Source: three-view drawing plus pictorial views. Frame: mm from the lowest corner of the part. Give positions to 0.01 mm unless a question says otherwise; leave off trailing zeros. Loops run counter-clockwise (first coordinate to the right, second up) from the corner with the lowest first, then second, coordinate; pieces in that order, holes last. Notation, with made-up numbers: (14.25, 47) -> (68.25, 47) arc R16 cw to (68.25, 52) -> close; hole circle Ø1 at (-36.75, 58). An arc over 180 degrees is marked (long way). Put each result on its own line as item: value.
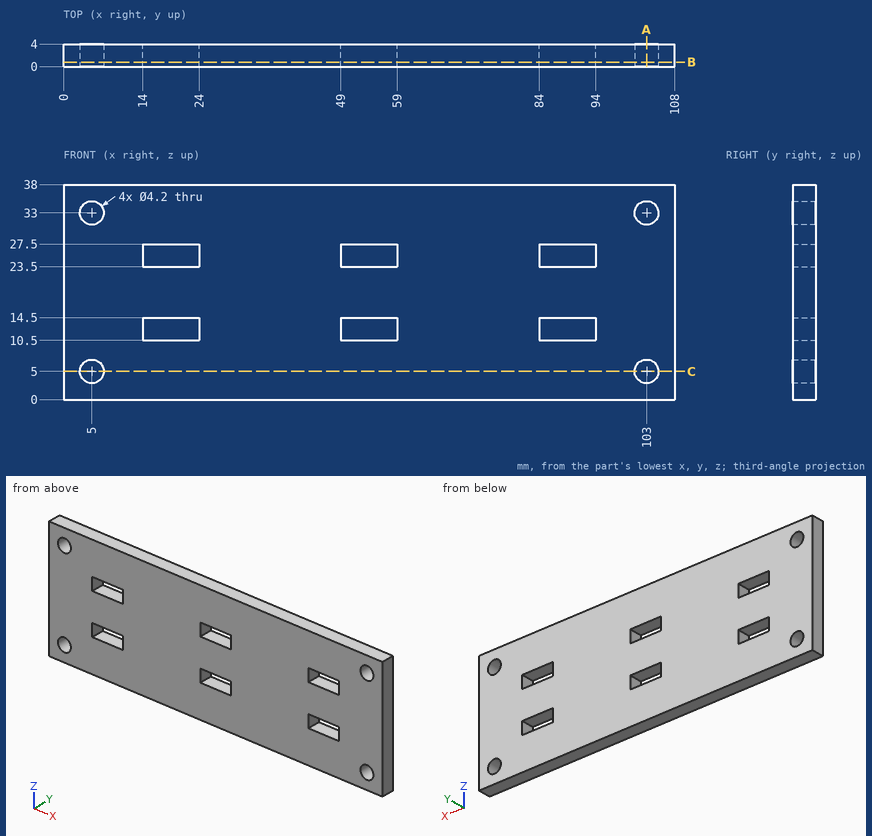
(1) Section B-B on y = 0.8. Give the number of separate pieces and of enclosed holes in the cut face, then the cut area to 3 significant figures.
Calculated:
separate pieces: 1
enclosed holes: 10
area: 3,810 mm²
(2) Section A-A on x = 103. Return loops of the section in (y, z), then the cut area to 3 significant figures.
Calculated:
outline: (0, 0) -> (4, 0) -> (4, 2.9) -> (0, 2.9) -> close; (0, 7.1) -> (4, 7.1) -> (4, 30.9) -> (0, 30.9) -> close; (0, 35.1) -> (4, 35.1) -> (4, 38) -> (0, 38) -> close
area: 118 mm²
(3) Line query: probe 1 along X at (y, z) = (3.15, 33); probe 2 along Z at (x, y) = (86.5, 3.05); probe 3 along X at (y, z) = (3.3, 11). Output: solid intervals per line, ascending. Write a range as from..to.
Calculated:
probe 1: x = 0..2.9, 7.1..100.9, 105.1..108
probe 2: z = 0..10.5, 14.5..23.5, 27.5..38
probe 3: x = 0..14, 24..49, 59..84, 94..108
(4) Section C-C on z = 5. Return loops of the section in (x, y).
Calculated:
outline: (0, 0) -> (2.9, 0) -> (2.9, 4) -> (0, 4) -> close; (7.1, 0) -> (100.9, 0) -> (100.9, 4) -> (7.1, 4) -> close; (105.1, 0) -> (108, 0) -> (108, 4) -> (105.1, 4) -> close
(5) First-contact query: P1, Ø2, axis at y = 3, z = 26, coming from the -X side. Flat tip, straight axial feed; report the tip coordinate or a pass-through.
Calculated:
P1: stops at x = 0
